Autodesk Inventor part; units mm, degrees
ref_plane "YZ Plane" through (0, 0, 0) normal (1, 0, 0) x (0, 1, 0)
ref_plane "XZ Plane" through (0, 0, 0) normal (0, 1, 0) x (-1, 0, 0)
ref_plane "XY Plane" through (0, 0, 0) normal (0, 0, 1) x (1, 0, 0)
sketch "Sketch1" plane through (0, 0, 0) normal (0, 1, 0) x (-1, 0, 0)
  line L0 (25.931, 23.0273) -> (-34.069, 23.0273)
  line L1 (-34.069, 23.0273) -> (-34.069, -23.9727)
  line L2 (-34.069, -23.9727) -> (25.931, -23.9727)
  line L3 (25.931, -23.9727) -> (25.931, 23.0273)
  point P0 (0, 0)
  dimension "d0" = 47
  dimension "d1" = 60
extrude "Extrusion1" add sketch "Sketch1" along normal blind 15
fillet "Fillet1" radius 2 4 edges at (34.069, 7.5, 23.0273) (34.069, 7.5, -23.9727) (-25.931, 7.5, 23.0273) (-25.931, 7.5, -23.9727)
sketch "Sketch2" plane through (0, 15, 0) normal (0, 1, 0) x (1, 0, 0)
  arc A0 (34.069, 21.9727) -> (32.069, 23.9727) centre (32.069, 21.9727) ccw
  line L0 (34.069, -20.2773) -> (0.569, -20.2773)
  line L1 (0.569, -20.2773) -> (0.569, -13.7773)
  line L2 (0.569, -13.7773) -> (-11.931, -13.7773)
  line L3 (-11.931, -13.7773) -> (-11.931, 20.9227)
  line L4 (34.069, -20.2773) -> (34.069, 20.9227)
  line L5 (34.069, -21.0273) -> (34.069, 21.9727)
  line L6 (-11.931, 20.9227) -> (34.069, 20.9227)
  line L7 (-23.931, -23.0273) -> (32.069, -23.0273)
  point P0 (0, 0)
  dimension "d5" = 33.5
  dimension "d6" = 41.2
  dimension "d7" = 2.75
  dimension "d8" = 6.5
  dimension "d9" = 46
extrude "Extrusion2" add sketch "Sketch2" along normal blind 8
fillet "Fillet2" radius 2 3 edges at (34.069, 19, -20.9227) (34.069, 19, 20.2773) (0.569, 19, 20.2773)
sketch "Sketch3" plane through (-11.931, 15, 13.7773) normal (0, 0, 1) x (1, 0, 0)
  line L0 (44, 8) -> (0, 8)
  line L1 (10, 8) -> (0, 8)
  line L2 (0, 0) -> (0, 8)
  line L3 (10, 8) -> (0, 3)
  line L4 (0, 0) -> (0, 8)
  line L5 (-12, 0) -> (44, 0)
  point P0 (11.931, -15)
  dimension "d13" = 10
  dimension "d14" = 3
extrude "Extrusion3" cut sketch "Sketch3" against normal blind 27
sketch "Sketch4" plane through (-11.931, 15, -20.9227) normal (0, 0, -1) x (-1, 0, 0)
  line L0 (-44, 8) -> (0, 8)
  line L1 (-6, 8) -> (0, 2)
  line L2 (0, 0) -> (0, 8)
  point P0 (-11.931, -15)
  dimension "d17" = 6
  dimension "d18" = 6
extrude "Extrusion4" cut sketch "Sketch4" against normal blind 5
sketch "Sketch5" plane through (0, 23, 0) normal (0, 1, 0) x (1, 0, 0)
  line L0 (-11.931, -13.7773) -> (-11.931, 13.2227)
  line L1 (-11.931, -11.0273) -> (-0.931, -11.0273)
  line L2 (-11.931, -8.0273) -> (-0.931, -8.0273)
  arc A0 (-0.931, -11.0273) -> (-0.931, -8.0273) centre (-0.931, -9.5273) ccw
  line L3 (-1.931, -13.7773) -> (-11.931, -13.7773)
  line L4 (-11.931, -2.0273) -> (-0.931, -2.0273)
  arc A1 (-0.931, -5.0273) -> (-0.931, -2.0273) centre (-0.931, -3.5273) ccw
  line L5 (-11.931, -5.0273) -> (-0.931, -5.0273)
  line L6 (-11.931, 3.9727) -> (-0.931, 3.9727)
  arc A2 (-0.931, 0.9727) -> (-0.931, 3.9727) centre (-0.931, 2.4727) ccw
  line L7 (-11.931, 0.9727) -> (-0.931, 0.9727)
  line L8 (-11.931, 9.9727) -> (-0.931, 9.9727)
  arc A3 (-0.931, 6.9727) -> (-0.931, 9.9727) centre (-0.931, 8.4727) ccw
  line L9 (-11.931, 6.9727) -> (-0.931, 6.9727)
  line L10 (-11.931, 15.9727) -> (-0.931, 15.9727)
  arc A4 (-0.931, 12.9727) -> (-0.931, 15.9727) centre (-0.931, 14.4727) ccw
  line L11 (-11.931, 12.9727) -> (-0.931, 12.9727)
  line L12 (-11.931, 15.9227) -> (-11.931, 13.2227)
  line L13 (-11.931, 15.9727) -> (-11.931, 12.9727)
  point P0 (0, 0)
  dimension "d21" = 3
  dimension "d22" = 1.5
  dimension "d23" = 2.75
  dimension "d24" = 11
  dimension "d27" = 6
extrude "Extrusion5" cut sketch "Sketch5" against normal blind 8
sketch "Sketch6" plane through (0, 23, 0) normal (0, 1, 0) x (1, 0, 0)
  line L0 (34.069, -18.2773) -> (34.069, 18.9227)
  line L1 (34.069, -13.2773) -> (31.569, -13.2773)
  line L2 (34.069, -10.2773) -> (31.569, -10.2773)
  arc A0 (31.569, -10.2773) -> (31.569, -13.2773) centre (31.569, -11.7773) ccw
  line L3 (2.569, -20.2773) -> (32.069, -20.2773)
  line L4 (34.069, -4.2773) -> (31.569, -4.2773)
  arc A1 (31.569, -4.2773) -> (31.569, -7.2773) centre (31.569, -5.7773) ccw
  line L5 (34.069, -7.2773) -> (31.569, -7.2773)
  line L6 (34.069, 1.7227) -> (31.569, 1.7227)
  arc A2 (31.569, 1.7227) -> (31.569, -1.2773) centre (31.569, 0.2227) ccw
  line L7 (34.069, -1.2773) -> (31.569, -1.2773)
  line L8 (34.069, 7.7227) -> (31.569, 7.7227)
  arc A3 (31.569, 7.7227) -> (31.569, 4.7227) centre (31.569, 6.2227) ccw
  line L9 (34.069, 4.7227) -> (31.569, 4.7227)
  line L10 (34.069, 13.7227) -> (31.569, 13.7227)
  arc A4 (31.569, 13.7227) -> (31.569, 10.7227) centre (31.569, 12.2227) ccw
  line L11 (34.069, 10.7227) -> (31.569, 10.7227)
  point P0 (0, 0)
  dimension "d35" = 1.5
  dimension "d36" = 3
  dimension "d37" = 2.5
  dimension "d38" = 7
  dimension "d41" = 6
extrude "Extrusion6" cut sketch "Sketch6" against normal blind 8
sketch "Sketch7" plane through (31.569, 23, 10.2773) normal (0, 0, 1) x (1, 0, 0)
  line L0 (-1.5, 0) -> (0, 0)
  line L1 (2.5, -8) -> (2.5, 0)
  line L2 (2.5, 0) -> (0, 0)
  line L3 (2.5, -4) -> (-1.5, 0)
  point P0 (-31.569, -23)
  dimension "d52" = 4
  dimension "d53" = 4
extrude "Extrusion7" cut sketch "Sketch7" against normal blind 22.5
extrude "Extrusion8" cut sketch "Sketch7" along normal blind 1.5
sketch "Sketch9" plane through (0, 15, 0) normal (0, 1, 0) x (1, 0, 0)
  line L0 (-14.681, 14.1727) -> (-23.681, 14.1727)
  line L1 (-23.681, 14.1727) -> (-23.681, -19.5273)
  line L2 (-23.681, -19.5273) -> (0.569, -19.5273)
  line L3 (0.569, -19.5273) -> (0.569, -13.7773)
  line L4 (0.569, -13.7773) -> (-17.931, -13.7773)
  line L5 (-17.931, -13.7773) -> (-17.931, 5.4227)
  line L6 (-17.931, 5.4227) -> (-14.681, 5.4227)
  line L7 (-14.681, 5.4227) -> (-14.681, 14.1727)
  line L8 (-25.931, 21.9727) -> (-25.931, -21.0273)
  line L9 (-23.931, -23.0273) -> (32.069, -23.0273)
  point P0 (0, 0)
  dimension "d58" = 9
  dimension "d59" = 5.75
  dimension "d60" = 24.25
  dimension "d61" = 33.7
  dimension "d62" = 8.75
  dimension "d63" = 2.25
  dimension "d64" = 3.5
  dimension "d65" = 5.75
extrude "Extrusion9" cut sketch "Sketch9" against normal blind 0.5
properties part number "Motor-controlling" material "Steel"
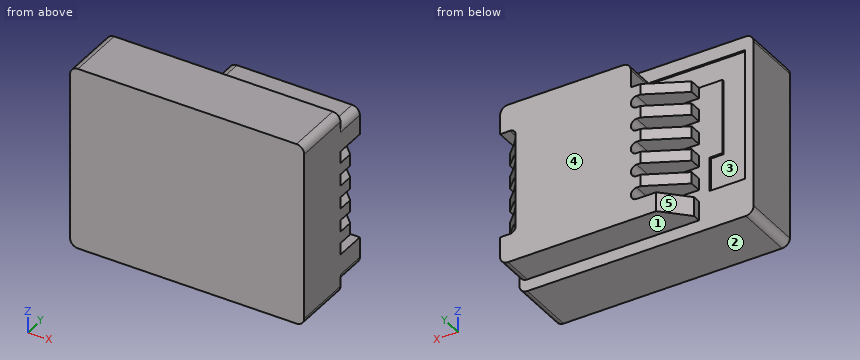
Source: CAD feature listing. Evaluate the final solid. Frame: model axes, mm. Face numbers are marked on the shaded views. A direction names the side the tool comes from. Coordinates: 2 decimals unless noted, no trailing zeros. Order: outer loops, then holes, each group sorted by start corner. A loop starts at its lowest first (then second) coordinate and runs counter-clockwise, first axis right, second up. Notation, with made-up numbers: (49.25, 89.25) - (99.25, 89.25) arc R10 ccw to (99.25, 102.25) - close; hole circle Ø2 at (9.5, 34.5). An arc over 180 degrees is marked (long way). One line per item, written item: value.
1) Reachability of the marked faces 1 and 2 from +Z, -Z, +X, -X, +Y, -Y: full face, straight path, thin tool, end or side. Return the list, or none.
Computed values:
face 1: -Z, +X, -X, +Y
face 2: -Z, +X, -X, +Y, -Y
2) Ray query, line 1 (Z direction, x = -2.5, y = 18); line 2 (Z direction, x = -21.5, y = 14.75); line 3 (Z direction, x = 27, y = 15.75). Return the intervals inside material, ascending. Write a range as [from, to].
Computed values:
line 1: z = [-20.92, -15.97], [-12.97, -9.97], [-6.97, -3.97], [-0.97, 2.03], [5.03, 8.03], [11.03, 13.78]
line 2: z = [-23.97, -14.17], [19.53, 23.03]
line 3: z = [-20.92, 20.28]
3) Cut plane A-A on x = 17. Output: boundary loops of the cut face in (y, z).
Computed values:
outline: (0, -23.97) - (15, -23.97) - (15, -20.92) - (23, -20.92) - (23, 20.28) - (15, 20.28) - (15, 23.03) - (0, 23.03) - close
4) Cut plane B-B on z = 9. Output: boundary loops of the cut face in (x, y).
Computed values:
outline: (-25.93, 0) - (34.07, 0) - (34.07, 19) - (30.07, 23) - (0.47, 23) - (0.47, 15) - (-17.93, 15) - (-17.93, 14.5) - (-23.68, 14.5) - (-23.68, 15) - (-25.93, 15) - close
5) Mould query, pull axis X, two halves, no side actions, for the marked faces 3, 4 and 5. Classes: released by +X, released by -X, zero draft, split by the parting line, or undercut.
Computed values:
face 3: undercut
face 4: zero draft
face 5: released by -X
6) Contact query for flat-ended pins moving along their axis: pin 1 (2 mm diameter, centred on x = 32.5, y = 18.5, fed in from -Z); pin 2 (1.5 mm diameter, centred on x = 31.5, z = -12.5, fed in from +Y); pin 3 (3 mm diameter, centred on x = -12, y = 20.5, fed in from +Z); pin 4 (6.5 mm diameter, centred on x = -4, y = 19, fed in from +Z). Output: stop coordinate, or through.
Computed values:
pin 1: stops at z = -20.92
pin 2: stops at y = 15
pin 3: passes through
pin 4: stops at z = 13.78
